The listing builds one solid part. Answer for the finished solid, in the listing's coordinates (mm). Face numbers are marked on the shaded views. A direction names the side the tool comes from. Round coordinates to 2 decimals unless told otherwise and drop trailing zeros. Write each loop counter-clockwise with the first axis right and the second up, starting at its lowest first coordinate (ties: lowest second). Pieces come first, ordered by that corner, then holes.
from build123d import *

# Parameters (mm, degrees)
F1_DEPTH = 60
F2_R     = 10
F3_DEPTH = 34.8
F4_W     = 15
F4_H     = 33.852546
F5_DEPTH = 10


with BuildPart() as f1:
    # F0 (on Front) → F1 (new body)
    with BuildSketch(Plane.XZ):
        Polygon((-60, 35), (-60, 0), (0, 0), (0, 10), (55, 10), (55, 35), (40, 35), (40, 25), (-45, 25), (-45, 35), align=None)
    extrude(amount=F1_DEPTH)

    # F2 (on Top) → F3 (cut)
    with BuildSketch(Plane.XY):
        with Locations((-26.186485, -28.806591)):
            Circle(F2_R)
        with Locations((21.658143, -28.806591)):
            Circle(F2_R)
    extrude(amount=F3_DEPTH, mode=Mode.SUBTRACT)

    # F4 (on face) → F5 (cut)
    with BuildSketch(Plane.XY.offset(35)):
        with Locations((47.5, -30)):
            Rectangle(F4_W, F4_H)
    extrude(amount=-F5_DEPTH, mode=Mode.SUBTRACT)


solid = f1.part
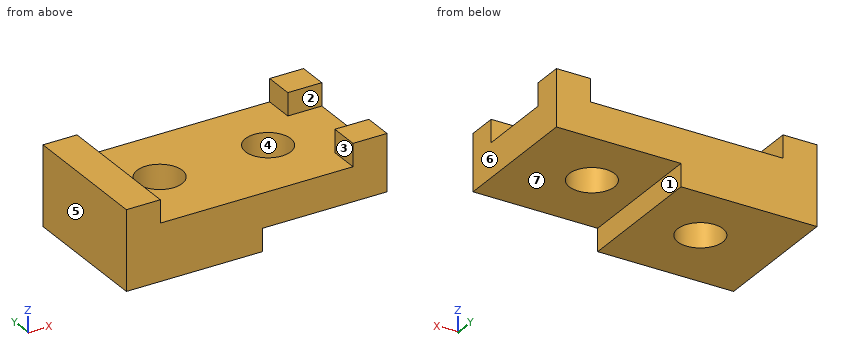
1. Straight lines are drawn through the part: line 1 along X through (y, z) = (-55, 29.5); line 2 along Y through (x, z) = (-26, 11); line 3 along X through (y, z) = (-33, 31). For each, find the intervals that lie inside material, in ascending order.
Geometry says:
line 1: x = -60 to -45, 40 to 55
line 2: y = -60 to -38.8, -18.81 to 0
line 3: x = -60 to -45
2. Section A-A on z = 31 is taken. Determine the outline of the cut face in (x, y), plus the area to 3 significant figures.
Geometry says:
outline: (-60, -60) - (-45, -60) - (-45, 0) - (-60, 0) - close; (40, -60) - (55, -60) - (55, -46.93) - (40, -46.93) - close; (40, -13.07) - (55, -13.07) - (55, 0) - (40, 0) - close
area: 1,290 mm2
3. A tool of negligible diameter and unlimited length cuts with its end or side. For the marked faces 1, 2 and 3, from which of +Z, -Z, +X, -X, +Y, -Y can it reach the whole face along a straight path? Write none if from no direction.
Geometry says:
face 1: -Z, +X, +Y, -Y
face 2: +Z, +X
face 3: +Z, +Y, -Y
4. For a pull along X with two mould halves and no side action, classify the marked faces 4, 5, 6 and 7 as released by +X, released by -X, zero draft, split by the parting line, or undercut.
Geometry says:
face 4: undercut
face 5: released by -X
face 6: released by +X
face 7: zero draft
5. Section D-D on y = -22 is taken. Determine the outline of the cut face in (x, z), plus the area to 3 significant figures.
Geometry says:
outline: (-60, 0) - (-33.51, 0) - (-33.51, 25) - (-45, 25) - (-45, 35) - (-60, 35) - close; (-18.86, 0) - (0, 0) - (0, 10) - (14.33, 10) - (14.33, 25) - (-18.86, 25) - close; (28.98, 10) - (55, 10) - (55, 25) - (28.98, 25) - close
area: 1,890 mm2
6. Given pin 1 (5 mm diameter, centred on y = -16, z = 29, fed in from +X); pin 2 (5 mm diameter, centred on x = 44.5, z = 31, fed in from +Y); pin 3 (3 mm diameter, centred on x = -35.5, y = -7.5, fed in from +Z), each flat-ended and moving along its own axis, determine where each tip first touches the part or whether it passes through.
Geometry says:
pin 1: stops at x = -45
pin 2: stops at y = 0
pin 3: stops at z = 25
7. Section C-C on x = 22.5 is taken. Determine the outline of the cut face in (y, z), plus the area to 3 significant figures.
Geometry says:
outline: (-60, 10) - (-38.77, 10) - (-38.77, 25) - (-60, 25) - close; (-18.84, 10) - (0, 10) - (0, 25) - (-18.84, 25) - close
area: 601 mm2
8. Section B-B on y = -15.5 is taken. Determine the outline of the cut face in (x, z).
Geometry says:
outline: (-60, 0) - (0, 0) - (0, 10) - (55, 10) - (55, 25) - (-45, 25) - (-45, 35) - (-60, 35) - close
